```python
from build123d import *

# Parameters (mm, degrees)
BOSS_EXTRUDE1_DEPTH  = 114.3
CUT_EXTRUDE1_START   = -1
SKETCH2_R            = 4
CUT_EXTRUDE1_DEPTH   = 7.35
M4_CLEARANCE_HOLE1_D = 4.8
FILLET1_R            = 4.7625
BOSS_EXTRUDE2_START  = 6.35
BOSS_EXTRUDE2_DEPTH  = 6.35
BOSS_EXTRUDE3_DEPTH  = 6.35
FILLET2_R            = 4.7625


with BuildPart() as part:
    # Sketch1 → Boss-Extrude1 (new body)
    with BuildSketch(Plane(origin=(0, 0, 0), x_dir=(0, 0, -1), z_dir=(1, 0, 0))):
        with BuildLine():
            Line((0, 22.225), (-4, 22.225))
            Line((-4, 22.225), (-4, 15.839643355))
            ThreePointArc((-3.999999999, 15.839643349), (-2.01539476, 16.212109221), (0, 16.336899995))
            Line((0, 16.336899995), (0, 17.4625))
            Line((0, 17.4625), (0, 22.225))
        make_face()
        with BuildLine():
            ThreePointArc((0, 16.336899995), (-2.01539476, 16.212109221), (-3.999999999, 15.839643349))
            ThreePointArc((-3.999999999, 15.839643349), (-16.336899991, 0), (-3.999999999, -15.839643349))
            ThreePointArc((-3.999999999, -15.839643349), (-2.01539476, -16.212109221), (0, -16.336899995))
            Line((0, -16.336899995), (0, -12.5269))
            ThreePointArc((0, -12.5269), (-12.361865073, -2.026700652), (-4, 11.871108778))
            ThreePointArc((-4, 11.871108778), (-2.026700652, 12.361865073), (0, 12.5269))
            Line((0, 12.5269), (0, 16.336899995))
        make_face()
        with BuildLine():
            ThreePointArc((0, -16.336899995), (-2.01539476, -16.212109221), (-3.999999999, -15.839643349))
            Line((-4, -15.839643355), (-4, -22.225))
            Line((-4, -22.225), (0, -22.225))
            Line((0, -22.225), (0, -17.4625))
            Line((0, -17.4625), (0, -16.336899995))
        make_face()
    extrude(amount=BOSS_EXTRUDE1_DEPTH)

    # Sketch2 → Cut-Extrude1 (cut)
    with BuildSketch(Plane.XY.offset(4).offset(CUT_EXTRUDE1_START)):
        with Locations(Location((19.05, -17.37595, 0), (0, 0, 157.413569734))):
            Circle(SKETCH2_R)
        with Locations(Location((57.15, -17.37595, 0), (0, 0, 157.413569734))):
            Circle(SKETCH2_R)
        with Locations(Location((95.25, -17.37595, 0), (0, 0, 157.413569734))):
            Circle(SKETCH2_R)
    cut_extrude1 = extrude(amount=CUT_EXTRUDE1_DEPTH, mode=Mode.SUBTRACT)

    # M4 Clearance Hole1 (through all)
    with Locations(Plane.XY.offset(4)):
        with Locations((19.05, -17.37595), (57.15, -17.37595), (95.25, -17.37595)):
            m4_clearance_hole1 = Hole(M4_CLEARANCE_HOLE1_D / 2)

    # Mirror1: Cut-Extrude1, M4 Clearance Hole1 across plane
    add(cut_extrude1.mirror(Plane.ZX), mode=Mode.SUBTRACT)
    add(m4_clearance_hole1.mirror(Plane.ZX), mode=Mode.SUBTRACT)

    # Fillet1
    fillet1_edges = [part.edges().sort_by_distance(p)[0] for p in [
        (0, 22.225, 2),
        (114.3, -22.225, 2),
    ]]
    fillet(fillet1_edges, radius=FILLET1_R)

    # Sketch8 → Boss-Extrude2 (add)
    with BuildSketch(Plane.ZY.offset(BOSS_EXTRUDE2_START)):
        with BuildLine():
            Line((3.999999999, 15.839643352), (4, 17.4625))
            Line((4, 17.4625), (0, 17.4625))
            Line((0, 17.4625), (0, 12.5269))
            ThreePointArc((0, 12.5269), (12.5269, 0), (0, -12.5269))
            Line((0, -12.5269), (0, -22.225))
            Line((0, -22.225), (4, -22.225))
            Line((4, -22.225), (3.999999999, -15.839643352))
            ThreePointArc((3.999999999, -15.839643352), (16.336899994, 0), (3.999999999, 15.839643352))
        make_face()
    extrude(amount=-BOSS_EXTRUDE2_DEPTH)

    # Sketch9 → Boss-Extrude3 (add)
    with BuildSketch(Plane(origin=(114.3, 0, 0), x_dir=(0, 0, -1), z_dir=(1, 0, 0))):
        with BuildLine():
            Line((-3.999999999, -15.839643352), (-4, -17.4625))
            Line((-4, -17.4625), (0, -17.4625))
            Line((0, -17.4625), (0, -12.5269))
            ThreePointArc((0, -12.5269), (-12.5269, 0), (0, 12.5269))
            Line((0, 12.5269), (0, 22.225))
            Line((0, 22.225), (-4, 22.225))
            Line((-4, 22.225), (-3.999999999, 15.839643352))
            ThreePointArc((-3.999999999, 15.839643352), (-16.336899994, 0), (-3.999999999, -15.839643352))
        make_face()
    extrude(amount=BOSS_EXTRUDE3_DEPTH)

    # Fillet2
    fillet2_edges = [part.edges().sort_by_distance(p)[0] for p in [
        (-6.35, 17.4625, 2),
        (-6.35, -22.225, 2),
        (120.65, -17.4625, 2),
        (120.65, 22.225, 2),
    ]]
    fillet(fillet2_edges, radius=FILLET2_R)


solid = part.part
```
Work out the finished part from the listing and answer in its coordinate system (mm). A direction names the side the tool comes from. Coordinates: 2 decimals unless noted, no trailing zeros. Write each loop counter-clockwise with the first axis right and the second up, starting at its lowest first coordinate (ties: lowest second). Pieces come first, ordered by that corner, then holes.
Q1. A cutting plane is placed at A-A, the plane x = 95.25. Give the vertices of the cut face in (y, z) (3 decimals), then the cut area to 3 significant figures.
Q2. Which of the six approach directions +Z, -Z, +X, -X, +Y, -Y give full straight-line access (tool end or side, diameter ignored) to faces 1 (the face through (18, 15, 3)), 2 (the face through (19.4, -15, 1.5))?
Q3. Find the intervals of material crossed by line 1 (Y direction, x = 19.05, z = 0.8) (3 decimals); line 2 (Y direction, x = 114, z = 7.75); line 3 (Z direction, x = 13, y = 0), in increasing order.
Q4. A cutting plane is placed at D-D, the plane x = 77.5. Give the vertices of the cut face in (y, z) (3 decimals), then the cut area to 3 significant figures.
Q5. A cutting plane is placed at B-B, the plane z = 1.5. State how many separate pieces and enclosed holes the cut face has, then the cut area to 3 significant figures.
Q6. Determine the mould class of faces 3 (the face through (-4.992, -20.793, 2.028)), 4 (the face through (120.65, 3.6, 12.4)), 5 (the face through (92.96, 16.66, 1.48)), 6 (the face through (119.292, 20.793, 2.028)) for opening direction Y: released by +Y, released by -Y, zero draft, split by the parting line, or undercut.
Q7. Each of these flat-tipped pins is pushed along its axis until it touches: pin 1 Ø0.5 at (x, z) = (-1, 2) entering from +Y; pin 2 Ø5 at (y, z) = (16, 8.5) entering from -X; pin 3 Ø4 at (x, y) = (57.15, 17.38) entering from +Z; pin 4 Ø8 at (x, z) = (8, 11) entering from +Y. Where does it stop, or does it pass through?
Q8. A cutting plane is placed at C-C, the plane y = -5.5. Give the vertices of the cut face in (x, z), then the cut area to 3 significant figures.
Findings below:
1. outline: (-22.225, 0) - (-19.776, 0) - (-19.776, 3) - (-21.376, 3) - (-21.376, 4) - (-22.225, 4) - close; (-14.976, 0) - (-12.527, 0) arc R12.527 cw to (12.527, 0) - (14.976, 0) - (14.976, 3) - (13.376, 3) - (13.376, 9.38) arc R16.337 ccw to (-13.376, 9.38) - (-13.376, 3) - (-14.976, 3) - close; (19.776, 0) - (22.225, 0) - (22.225, 4) - (21.376, 4) - (21.376, 3) - (19.776, 3) - close
1. area: 161 mm2
2. face 1: +Z
2. face 2: +Z, -Z
3. line 1: y = -22.225 to -19.776, -14.976 to -12.501, 12.501 to 14.976, 19.776 to 22.225
3. line 2: y = -14.38 to -9.84, 9.84 to 14.38
3. line 3: z = 12.53 to 16.34
4. outline: (-22.225, 0) - (-12.527, 0) arc R12.527 cw to (12.527, 0) - (22.225, 0) - (22.225, 4) - (15.84, 4) arc R16.337 ccw to (-15.84, 4) - (-22.225, 4) - close
4. area: 221 mm2
5. separate pieces: 2
5. enclosed holes: 6
5. area: 2,290 mm2
6. face 3: released by -Y
6. face 4: zero draft
6. face 5: undercut
6. face 6: released by +Y
7. pin 1: stops at y = 17.46
7. pin 2: stops at x = -6.28
7. pin 3: passes through
7. pin 4: stops at y = 14.76
8. outline: (-6.35, 11.25) - (120.65, 11.25) - (120.65, 15.38) - (-6.35, 15.38) - close
8. area: 524 mm2
